Here's how the part is built. I have some questions about the finished solid (model axes, mm). A direction names the side the tool comes from. Round coordinates to 2 decimals unless told otherwise and drop trailing zeros. Write each loop counter-clockwise with the first axis right and the second up, starting at its lowest first coordinate (ties: lowest second). Pieces come first, ordered by that corner, then holes. Notation, with made-up numbers: (3, 3.5) -> (62, 3.5) arc R19 ccw to (62, 26.5) -> close; hole circle Ø9 at (36.5, 0.5). An arc over 180 degrees is marked (long way). Answer in a Markdown table with one row per item. Add a question column.
from build123d import *

# Parameters (mm, degrees)
SKETCH1_R           = 34.1376
BOSS_EXTRUDE1_DEPTH = 6.35
SKETCH2_R           = 31.0896
CUT_EXTRUDE3_DEPTH  = 3.175
SKETCH3_R           = 6.35
CUT_EXTRUDE4_DEPTH  = 3.175
SKETCH3_3_R         = 6.35
SKETCH3_3_R_2       = 1.778
CUT_EXTRUDE5_DEPTH  = 3.175
SKETCH6_R           = 1.778
CUT_EXTRUDE6_DEPTH  = 3.175
SKETCH8_R           = 1.778
CUT_EXTRUDE7_DEPTH  = 3.175


with BuildPart() as part:
    # Sketch1 → Boss-Extrude1 (new body)
    with BuildSketch(Plane(origin=(0, 0, 0), x_dir=(1, 0, 0), z_dir=(0, 1, 0))):
        with Locations(Location((0, 0, 0), (0, 0, 270))):
            Circle(SKETCH1_R)
    extrude(amount=BOSS_EXTRUDE1_DEPTH)

    # Sketch2 → Cut-Extrude3 (cut)
    with BuildSketch(Plane(origin=(0, 6.35, 0), x_dir=(1, 0, 0), z_dir=(0, 1, 0))):
        with Locations(Location((0, 0, 0), (0, 0, 270))):
            Circle(SKETCH2_R)
    extrude(amount=-CUT_EXTRUDE3_DEPTH, mode=Mode.SUBTRACT)

    # Sketch3 → Cut-Extrude4 (cut)
    with BuildSketch(Plane(origin=(0, 3.175, 0), x_dir=(1, 0, 0), z_dir=(0, 1, 0))):
        with Locations(Location((0, 0, 0), (0, 0, 270))):
            Circle(SKETCH3_R)
    extrude(amount=-CUT_EXTRUDE4_DEPTH, mode=Mode.SUBTRACT)

    # Sketch3_3 → Cut-Extrude5 (cut)
    with BuildSketch(Plane(origin=(0, 3.175, 0), x_dir=(1, 0, 0), z_dir=(0, 1, 0))):
        with Locations(Location((0, 0, 0), (0, 0, 270))):
            Circle(SKETCH3_3_R)
        with Locations(Location((25.4, 0, 0), (0, 0, 270))):
            Circle(SKETCH3_3_R_2)
        with Locations(Location((17.960512242, 17.960512242, 0), (0, 0, 270))):
            Circle(SKETCH3_3_R_2)
        with Locations(Location((0, 25.4, 0), (0, 0, 270))):
            Circle(SKETCH3_3_R_2)
        with Locations(Location((-17.960512242, 17.960512242, 0), (0, 0, 270))):
            Circle(SKETCH3_3_R_2)
        with Locations(Location((-25.4, 0, 0), (0, 0, 270))):
            Circle(SKETCH3_3_R_2)
        with Locations(Location((-17.960512242, -17.960512242, 0), (0, 0, 270))):
            Circle(SKETCH3_3_R_2)
        with Locations(Location((0, -25.4, 0), (0, 0, 270))):
            Circle(SKETCH3_3_R_2)
        with Locations(Location((17.960512242, -17.960512242, 0), (0, 0, 270))):
            Circle(SKETCH3_3_R_2)
    extrude(amount=-CUT_EXTRUDE5_DEPTH, mode=Mode.SUBTRACT)

    # Sketch6 → Cut-Extrude6 (cut)
    with BuildSketch(Plane(origin=(0, 3.175, 0), x_dir=(1, 0, 0), z_dir=(0, 1, 0))):
        with Locations(Location((0, 19.05, 0), (0, 0, 270))):
            Circle(SKETCH6_R)
        with Locations(Location((-13.470384182, 14.10896611, 0), (0, 0, 270))):
            Circle(SKETCH6_R)
        with Locations(Location((-19.05, 0, 0), (0, 0, 270))):
            Circle(SKETCH6_R)
        with Locations(Location((-13.470384182, -13.470384182, 0), (0, 0, 270))):
            Circle(SKETCH6_R)
        with Locations(Location((0, -19.05, 0), (0, 0, 270))):
            Circle(SKETCH6_R)
        with Locations(Location((13.470384182, -13.470384182, 0), (0, 0, 270))):
            Circle(SKETCH6_R)
        with Locations(Location((19.05, 0, 0), (0, 0, 270))):
            Circle(SKETCH6_R)
        with Locations(Location((13.470384182, 13.470384182, 0), (0, 0, 270))):
            Circle(SKETCH6_R)
    extrude(amount=-CUT_EXTRUDE6_DEPTH, mode=Mode.SUBTRACT)

    # Sketch8 → Cut-Extrude7 (cut)
    with BuildSketch(Plane(origin=(0, 3.175, 0), x_dir=(1, 0, 0), z_dir=(0, 1, 0))):
        with Locations(Location((9.779, 0, 0), (0, 0, 270))):
            Circle(SKETCH8_R)
        with Locations(Location((6.914797213, 6.914797213, 0), (0, 0, 270))):
            Circle(SKETCH8_R)
        with Locations(Location((0, 9.779, 0), (0, 0, 270))):
            Circle(SKETCH8_R)
        with Locations(Location((-6.914797213, 6.914797213, 0), (0, 0, 270))):
            Circle(SKETCH8_R)
        with Locations(Location((-9.779, 0, 0), (0, 0, 270))):
            Circle(SKETCH8_R)
        with Locations(Location((-6.914797213, -6.914797213, 0), (0, 0, 270))):
            Circle(SKETCH8_R)
        with Locations(Location((0, -9.779, 0), (0, 0, 270))):
            Circle(SKETCH8_R)
        with Locations(Location((6.914797213, -6.914797213, 0), (0, 0, 270))):
            Circle(SKETCH8_R)
    extrude(amount=-CUT_EXTRUDE7_DEPTH, mode=Mode.SUBTRACT)


solid = part.part
Item 1: If we section it at C-C on y = 5: Please give me the cut outline in (x, z).
Item 2: On a 3-axis mill with a long thin cutter (end or side, diameter ignored), from which of +Z, -Z, +X, -X, +Y, -Y can I reach the whole of each face in a straight line? I mean faces 4 (the cylindrical face through (30.825, 4.785, -4.047)), 5 (the cylindrical face through (-23.637, 1.61, -0.231)). Say none if no direction works.
Item 3: I need wall thicknesses on line 1 along X through (y, z) = (1.8, 19.05); line 2 along Z through (x, y) = (17.5, 2); line 3 along Y through (x, z) = (-22.5, -12.5) (3 decimals). Which ranges of each line are inside material? Lowest first, please. Write a range as from..to.
Item 4: If we section it at B-B on z = 12.5: Please give me the cut outline in (x, y) (3 decimals), then the cut area to 3 significant figures.
Item 5: If we section it at D-D on z = 25.4: Please give me the cut outline in (x, y) (3 decimals), then the cut area to 3 significant figures.
Item 6: If we section it at A-A on x = 25.4: Please give me the cut outline in (y, z) (3 decimals), then the cut area to 3 significant figures.
Item 7: If we mould it in two halves opening along X, with no side actions, what happens to faces 1 (the flat face through (-15, 6.35, 28)), 2 (the cylindrical face through (7.45, 1.61, -5.22)), 3 (the cylindrical face through (16.383, 1.61, 18.781))? For each: pulls with the +X half, pulls with the -X half, needs draft (parallel to the pull), parting line crosses it, or undercut.
Item 8: For P1, Ø1, axis at x = 24.5, z = -14.5, coming from the +Y side (3 decimals); P2, Ø3, axis at x = -13.47, z = 13.47, coming from the -Y side; P3, Ø1.5, axis at y = 3, z = 20.5, coming from the -X side; P4, Ø3, axis at y = 5, z = 1.5, coming from the +X side, each with a flat end and sliding along its axis, tell me the tip position at first contact or that it passes through.
Results list:
| question | item | result |
|---|---|---|
| 1 | outline | circle Ø68.28 at (0, 0); hole circle Ø62.18 at (0, 0) |
| 2 | face 4 | +Y |
| 2 | face 5 | +Y, -Y |
| 3 | line 1 | -28.33..-19.37, -16.56..-1.78, 1.78..16.56, 19.37..28.33 |
| 3 | line 2 | -29.31..-19.68, -16.24..-0.87, 0.87..16.24, 19.68..29.31 |
| 3 | line 3 | 0..3.175 |
| 4 | outline | (-31.767, 0) -> (-14.96, 0) -> (-14.96, 3.175) -> (-28.466, 3.175) -> (-28.466, 6.35) -> (-31.767, 6.35) -> close; (-11.981, 0) -> (11.981, 0) -> (11.981, 3.175) -> (-11.981, 3.175) -> close; (14.96, 0) -> (31.767, 0) -> (31.767, 6.35) -> (28.466, 6.35) -> (28.466, 3.175) -> (14.96, 3.175) -> close |
| 4 | area | 204 mm² |
| 5 | outline | (-22.808, 0) -> (-1.778, 0) -> (-1.778, 3.175) -> (-17.928, 3.175) -> (-17.928, 6.35) -> (-22.808, 6.35) -> close; (1.778, 0) -> (22.808, 0) -> (22.808, 6.35) -> (17.928, 6.35) -> (17.928, 3.175) -> (1.778, 3.175) -> close |
| 5 | area | 165 mm² |
| 6 | outline | (0, -22.808) -> (6.35, -22.808) -> (6.35, -17.928) -> (3.175, -17.928) -> (3.175, -1.778) -> (0, -1.778) -> close; (0, 1.778) -> (3.175, 1.778) -> (3.175, 17.928) -> (6.35, 17.928) -> (6.35, 22.808) -> (0, 22.808) -> close |
| 6 | area | 165 mm² |
| 7 | face 1 | needs draft |
| 7 | face 2 | undercut |
| 7 | face 3 | undercut |
| 8 | P1 | y = 3.175 |
| 8 | P2 | through |
| 8 | P3 | x = -27.84 |
| 8 | P4 | x = 34.14 |
